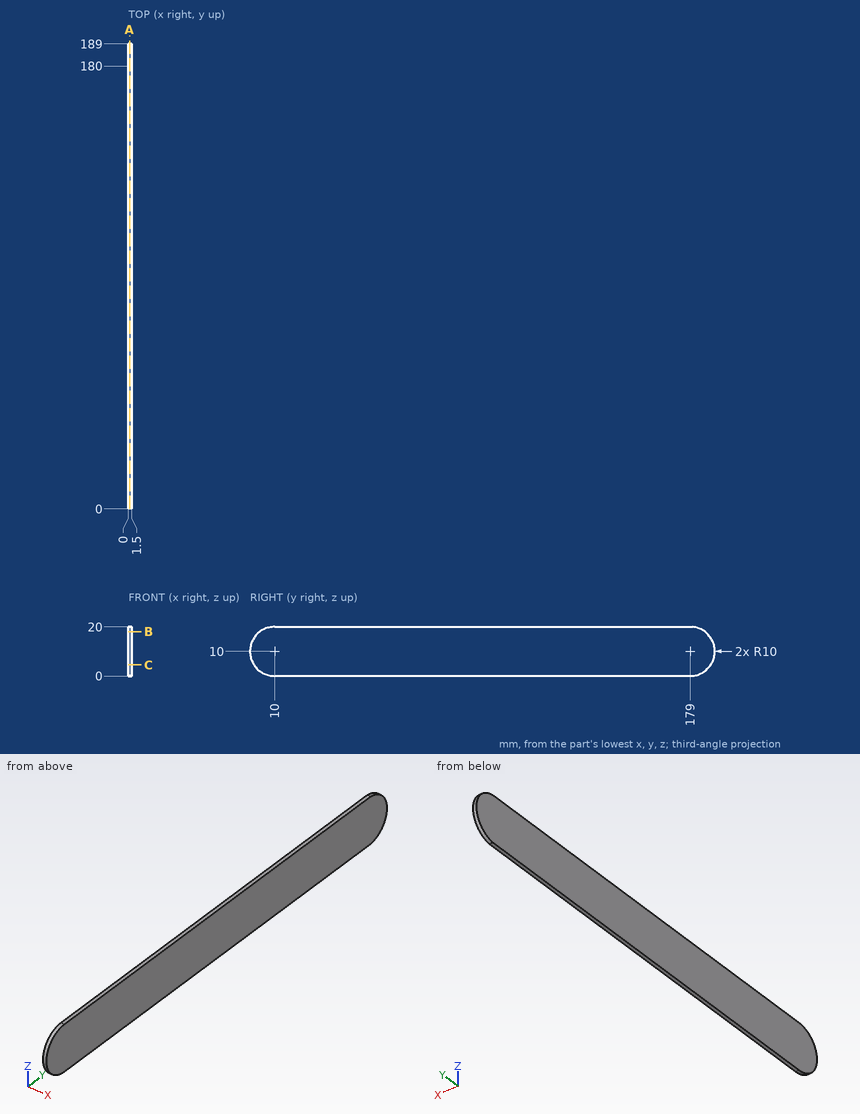
Can you work these out from the drawing? Everything is in mm from the part's minimum corner. Round coordinates to 2 decimals unless told otherwise and drop trailing zeros. Loops run counter-clockwise (first coordinate to the right, second up) from the corner with the lowest first, then second, coordinate; pieces in that order, holes last. Notation, with made-up numbers: (21.5, -14.5) - (49.5, -14.5) arc R14 cw to (49.5, -10.5) - close; hole circle Ø4 at (65.25, -39). An arc over 180 degrees is marked (long way). Answer in a Markdown table with one row per item. Add a question column.
(1) I need wall thicknesses on line 1 along Y through (x, z) = (0.3, 9.25); line 2 along Y through (x, z) = (1.25, 6.25). Which ranges of each line are inside material? Lowest first, please.
(2) If we section it at C-C (z = 4.5): Please give me the cut outline in (x, y).
(3) If we section it at A-A (x = 0.55): Please give me the cut outline in (y, z), plus the area to 3 significant figures.
(4) I'm going to push a flat-ended pin straight in: pin 1 (2 mm diameter, centred on y = 159.5, z = 10.5, fed in from -X). Where does the tip first touch, or does it pass through?
(5) If we section it at B-B (z = 18): Please give me the cut outline in (x, y).
Model answer:
| question | item | result |
|---|---|---|
| 1 | line 1 | y = 0.03 to 188.97 |
| 1 | line 2 | y = 0.73 to 188.27 |
| 2 | outline | (0, 1.65) - (1.5, 1.65) - (1.5, 187.35) - (0, 187.35) - close |
| 3 | outline | (10, 0) - (180, 0) - (180, 0.05) arc R10 ccw to (180, 19.95) - (180, 20) - (10, 20) arc R10 ccw to start |
| 3 | area | 3,690 mm² |
| 4 | pin 1 | stops at x = 0 |
| 5 | outline | (0, 4) - (1.5, 4) - (1.5, 185) - (0, 185) - close |
